Could you check a few things on this model? Use its own coordinates, in mm. A direction names the side the tool comes from. Round coordinates to 2 decimals unless told otherwise and drop trailing zeros. Write each loop counter-clockwise with the first axis right and the second up, starting at its lowest first coordinate (ties: lowest second). Pieces come first, ordered by that corner, then holes. Notation, with made-up numbers: (-28, 58.25) -> (-21, 58.25) arc R24 ccw to (-21, 81.25) -> close; hole circle Ø9 at (8.5, 46). An arc over 180 degrees is marked (long way). One line per question, with ' | ' between items. Start each with the question number.
1. Imagine slicing it at B-B, the plane y = 4.5. List the corners of the cut face in (x, z) for me, and give its area (3 significant figures).
2. For pin 1 Ø1.5 at (x, z) = (-1.5, 6.5) entering from +Y; pin 2 Ø3 at (y, z) = (-3.5, 5.5) entering from +X; pin 3 Ø1 at (x, y) = (-2.5, 6.5) entering from -Z, each with a flat end and sliding along its axis, tell me the tip position at first contact or that it passes through.
3. If I drill on line 1 along Y through (x, z) = (-5, -1.25); line 2 along X through (y, z) = (-5.5, 7); line 3 along X through (y, z) = (-4.5, 1.75), over which ranges is the centre line in solid material (lowest first)? Write a range as [from, to].
4. For faces 1 (the flat face through (5, -7, 0)), 2 (the flat face through (2.1, 0, 2.4)), which set-ups out of +Z, -Z, +X, -X, +Y, -Y let a thin tool reach every point of the face, with its end or its side?
5. Imagine slicing it at A-A, the plane z = 0. List the corners of the cut face in (x, y) for me.
Autodesk Inventor part; units mm, degrees
ref_plane "YZ Plane" through (0, 0, 0) normal (1, 0, 0) x (0, 1, 0)
ref_plane "XZ Plane" through (0, 0, 0) normal (0, 1, 0) x (-1, 0, 0)
ref_plane "XY Plane" through (0, 0, 0) normal (0, 0, 1) x (1, 0, 0)
sketch "Sketch1" plane through (0, 0, 0) normal (0, 1, 0) x (-1, 0, 0)
  circle A0 centre (0, 0) radius 3
  dimension "d0" = 6
extrude "Extrusion1" add sketch "Sketch1" along normal blind 20
sketch "Sketch2" plane through (0, 0, 0) normal (0, -1, 0) x (1, 0, 0)
  circle A0 centre (0, 0) radius 10
  dimension "d3" = 20
extrude "Extrusion2" add sketch "Sketch2" along normal blind 7
chamfer "Chamfer1" distance 1 angle 45 1 edges at (3, 20, 0)
sketch "Sketch3" plane through (0, -7, 0) normal (0, -1, 0) x (1, 0, 0)
  line L0 (-1, 12.4438) -> (1, 12.4438)
  line L1 (1, 12.4438) -> (1, -12.4438)
  line L2 (1, -12.4438) -> (-1, -12.4438)
  line L3 (-1, -12.4438) -> (-1, 12.4438)
  line L4 (-1, 12.4438) -> (1, -12.4438) construction
  line L5 (1, 12.4438) -> (-1, -12.4438) construction
  point P0 (0, 0)
  dimension "d9" = 2
extrude "Extrusion3" cut sketch "Sketch3" against normal blind 2
fillet "Fillet1" radius 0.7 13 edges at (-10, -7, 0) (7.4162, -7, -6.7082) (7.4162, -7, 6.7082) (1, -7, 0) (1, -6, -9.9499) (1, -6, 9.9499) (1, -5, 0) (0, -5, -10) (0, -5, 10) (-1, -5, 0) (-1, -6, -9.9499) (-1, -6, 9.9499) (-1, -7, 0)
thread "Thread1"
properties part number "M6x1 Feet" material "Stainless Steel"
Geometry results:
1) outline: circle Ø6 at (0, 0) | area: 28.3 mm2
2) pin 1: stops at y = 0 | pin 2: stops at x = 9.17 | pin 3: stops at z = -2.24
3) line 1: y = [-7, 0] | line 2: x = [-7.14, -0.97], [0.97, 7.14] | line 3: x = [-9.85, 9.85]
4) face 1: +Z, -Z, +X, -X, -Y | face 2: +Y
5) outline: (-10, -6.3) arc R0.7 ccw to (-9.3, -7) -> (-1.7, -7) arc R0.7 ccw to (-1, -6.3) -> (-1, -5.7) arc R0.7 cw to (-0.3, -5) -> (0.3, -5) arc R0.7 cw to (1, -5.7) -> (1, -6.3) arc R0.7 ccw to (1.7, -7) -> (9.3, -7) arc R0.7 ccw to (10, -6.3) -> (10, 0) -> (3, 0) -> (3, 19) -> (2, 20) -> (-2, 20) -> (-3, 19) -> (-3, 0) -> (-10, 0) -> close
